Geometry: final body of the model. Coordinates: model frame, mm. Coordinates: 2 decimals unless noted, no trailing zeros. Loops run counter-clockwise (first coordinate to the right, second up) from the corner with the lowest first, then second, coordinate; pieces in that order, holes last. Notation, with made-up numbers: (87.25, 23.5) - (144.25, 23.5) arc R20 ccw to (144.25, 28.5) - close; hole circle Ø10 at (55, 85). An arc over 180 degrees is marked (long way). Write each question's results on one line, items separated by ' | '. Start each with the question number.
from build123d import *

# Parameters (mm, degrees)
BOSS_EXTRUDE1_DEPTH = 25
SKETCH2_R           = 14.285
CUT_EXTRUDE1_DEPTH  = 321.507410211


with BuildPart() as part:
    # Sketch1 → Boss-Extrude1 (new body)
    with BuildSketch(Plane(origin=(0, 0, 0), x_dir=(1, 0, 0), z_dir=(0, 1, 0))):
        with BuildLine():
            Line((0, 0), (0, 90))
            ThreePointArc((0, 90), (5.857864376, 104.142135624), (20, 110))
            Line((20, 110), (280, 110))
            ThreePointArc((280, 110), (294.142135624, 104.142135624), (300, 90))
            Line((300, 90), (300, 0))
            Line((300, 0), (300, -90))
            ThreePointArc((300, -90), (294.142135624, -104.142135624), (280, -110))
            Line((280, -110), (20, -110))
            ThreePointArc((20, -110), (5.857864376, -104.142135624), (0, -90))
            Line((0, -90), (0, 0))
        make_face()
    extrude(amount=BOSS_EXTRUDE1_DEPTH)

    # Sketch2 → Cut-Extrude1 (cut, through all)
    with BuildSketch(Plane(origin=(0, 0, 0), x_dir=(0, 0, -1), z_dir=(1, 0, 0))):
        Circle(SKETCH2_R)
    extrude(amount=CUT_EXTRUDE1_DEPTH, mode=Mode.SUBTRACT)


solid = part.part
1) Material intervals for line 1 (Z direction, x = 184.5, y = 4.75); line 2 (Z direction, x = 98, y = 11.75); line 3 (Y direction, x = 131.5, z = -9), sorted ascending. Write a range as [from, to].
2) Section query A-A on z = 0. Output: boundary loops of the cut face in (x, y) (3 decimals), and give its area (3 significant figures).
3) Pin query (flat end, axial travel): pin 1 Ø4 at (x, z) = (245, -10.5) entering from -Y. Return the tip coordinate at first contact, or that it passes through.
4) Section query B-B on x = 103.5. Output: boundary loops of the cut face in (y, z) (3 decimals), and give its area (3 significant figures).
5) Pull-direction query (Z, two-part tool) for faces 1 (the flat face through (152, 25, -2)), 2 (the flat face through (148, 12, -110)), 3 (the cylindrical face through (147.9, 14.28, -0.31)); classes: released by +Z, released by -Z, zero draft, split by the parting line, or undercut.
Returned:
1) line 1: z = [-110, -13.47], [13.47, 110] | line 2: z = [-110, -8.12], [8.12, 110] | line 3: y = [11.09, 25]
2) outline: (0, 14.285) - (300, 14.285) - (300, 25) - (0, 25) - close | area: 3,210 mm²
3) pin 1: stops at y = 6.91
4) outline: (0, -110) - (25, -110) - (25, 110) - (0, 110) - (0, 14.285) arc R14.285 cw to (0, -14.285) - close | area: 5,180 mm²
5) face 1: zero draft | face 2: released by -Z | face 3: undercut
